```python
from build123d import *

# Parameters (mm, degrees)
SKETCH1_W           = 13.5
SKETCH1_H           = 29
BOSS_EXTRUDE1_DEPTH = 2
BOSS_EXTRUDE2_DEPTH = 56
BOSS_EXTRUDE3_DEPTH = 2
BOSS_EXTRUDE6_DEPTH = 23
SKETCH7_R           = 4.875
CUT_EXTRUDE2_DEPTH  = 6
BOSS_EXTRUDE7_REACH = 60
BOSS_EXTRUDE8_DEPTH = 6
CUT_EXTRUDE11_DEPTH = 5
SKETCH17_R          = 0.75
CUT_EXTRUDE13_DEPTH = 6
SKETCH18_R          = 6.425
CUT_EXTRUDE14_DEPTH = 6
SKETCH8_R           = 4.875
SKETCH8_R_2         = 2.775
CUT_EXTRUDE20_DEPTH = 20
SKETCH5_R           = 2.775
CUT_EXTRUDE21_DEPTH = 26
SKETCH19_R          = 2.775
CUT_EXTRUDE22_DEPTH = 26


with BuildPart() as part:
    # Sketch1 → Boss-Extrude1 (new body)
    with BuildSketch(Plane.XY):
        Polygon((23.484890655, 4.171572875), (0.484890655, 27.171572875), (0.484890655, -37.500000005), (23.484890655, -37.500000005), align=None)
        with Locations((11.635259587, -14.642279086)):
            Rectangle(SKETCH1_W, SKETCH1_H, mode=Mode.SUBTRACT)
        Polygon((23.484890655, 4.171572875), (23.484890655, -37.500000005), (0.484890655, -37.500000005), (0.484890655, -39.5), (25.484890655, -39.5), (25.484890655, 5), (0.484890655, 30), (0.484890655, 27.171572875), align=None)
    extrude(amount=BOSS_EXTRUDE1_DEPTH)

    # Sketch2 → Boss-Extrude2 (add)
    with BuildSketch(Plane.XY.offset(2)):
        Polygon((23.484890655, -37.500000005), (0.484890655, -37.500000005), (0.484890655, -39.5), (25.484890655, -39.5), (25.484890655, 5), (0.484890655, 30), (0.484890655, 27.171572875), (23.484890655, 4.171572875), align=None)
    extrude(amount=BOSS_EXTRUDE2_DEPTH)

    # Sketch3 → Boss-Extrude3 (add)
    with BuildSketch(Plane.XY.offset(58)):
        Polygon((25.484890655, 5), (0.484890655, 30), (0.484890655, -39.5), (25.484890655, -39.5), align=None)
    extrude(amount=BOSS_EXTRUDE3_DEPTH)

    # Sketch6 → Boss-Extrude6 (add)
    with BuildSketch(Plane.ZY.offset(-23.484890655)):
        with BuildLine():
            Line((37, -37.500000005), (37, -31.5))
            ThreePointArc((37, -31.5), (30, -24.5), (23, -31.5))
            Line((23, -31.5), (23, -37.500000005))
            Line((23, -37.500000005), (37, -37.500000005))
        make_face()
    extrude(amount=BOSS_EXTRUDE6_DEPTH)

    # Sketch7 → Cut-Extrude2 (cut)
    with BuildSketch(Plane(origin=(25.484890655, 0, 0), x_dir=(0, 0, -1), z_dir=(1, 0, 0))):
        with Locations((-30, -31.5)):
            Circle(SKETCH7_R)
    extrude(amount=-CUT_EXTRUDE2_DEPTH, mode=Mode.SUBTRACT)

    # Sketch9 → Boss-Extrude7 (add, up to next)
    with BuildSketch(Plane.XY.offset(2), mode=Mode.PRIVATE) as boss_extrude7_sk1:
        Polygon((0.484890655, 27.171572875), (17.541784111, 10.114679419), (0.484890655, 10.114679419), align=None)
    boss_extrude7_tool1 = extrude(boss_extrude7_sk1.sketch, amount=BOSS_EXTRUDE7_REACH, mode=Mode.PRIVATE) - part.part
    add(boss_extrude7_tool1.solids().sort_by_distance((6.170522, 15.800311, 2))[0])

    # Sketch14 → Boss-Extrude8 (add)
    with BuildSketch(Plane(origin=(0, 0, 58), x_dir=(-1, 0, 0), z_dir=(0, 0, -1))):
        Polygon((-17.541784111, 10.114679419), (-0.484890655, 10.114679419), (-0.484890655, -37.500000005), (-23.484890655, -37.500000005), (-23.484890655, 4.171572875), align=None)
    extrude(amount=BOSS_EXTRUDE8_DEPTH)

    # Sketch15 → Cut-Extrude11 (cut)
    with BuildSketch(Plane.XY.offset(60)):
        with BuildLine():
            Line((9.606797633, -3.100018288), (5.995686967, -10.67958818))
            ThreePointArc((5.995686967, -10.67958818), (5.371033475, -13.44302904), (5.995686967, -16.206469901))
            Line((5.995686967, -16.206469901), (9.606797633, -23.786039793))
            ThreePointArc((9.606797633, -23.786039793), (11.796033475, -25.16802904), (13.985269316, -23.786039793))
            Line((13.985269316, -23.786039793), (17.596379983, -16.206469901))
            ThreePointArc((17.596379983, -16.206469901), (18.221033475, -13.44302904), (17.596379983, -10.67958818))
            Line((17.596379983, -10.67958818), (13.985269316, -3.100018288))
            ThreePointArc((13.985269316, -3.100018288), (11.796033475, -1.71802904), (9.606797633, -3.100018288))
        make_face()
    extrude(amount=-CUT_EXTRUDE11_DEPTH, mode=Mode.SUBTRACT)

    # Sketch17 → Cut-Extrude13 (cut)
    with BuildSketch(Plane.XY.offset(55)):
        with Locations((11.796033475, -4.14302904)):
            Circle(SKETCH17_R)
        with Locations((11.796033475, -22.74302904)):
            Circle(SKETCH17_R)
    extrude(amount=-CUT_EXTRUDE13_DEPTH, mode=Mode.SUBTRACT)

    # Sketch18 → Cut-Extrude14 (cut)
    with BuildSketch(Plane.XY.offset(55)):
        with Locations((11.796033475, -13.44302904)):
            Circle(SKETCH18_R)
    extrude(amount=-CUT_EXTRUDE14_DEPTH, mode=Mode.SUBTRACT)

    # Sketch8 → Cut-Extrude20 (cut)
    with BuildSketch(Plane(origin=(25.484890655, 0, 0), x_dir=(0, 0, -1), z_dir=(1, 0, 0))):
        with Locations((-50, 18)):
            Circle(SKETCH8_R)
        with Locations((-50, 18)):
            Circle(SKETCH8_R_2, mode=Mode.SUBTRACT)
        with Locations((-10, 18)):
            Circle(SKETCH8_R)
        with Locations((-10, 18)):
            Circle(SKETCH8_R_2, mode=Mode.SUBTRACT)
    extrude(amount=-CUT_EXTRUDE20_DEPTH, mode=Mode.SUBTRACT)

    # Sketch5 → Cut-Extrude21 (cut, through all)
    with BuildSketch(Plane(origin=(25.484890655, 0, 0), x_dir=(0, 0, -1), z_dir=(1, 0, 0))):
        with Locations((-30, -31.5)):
            Circle(SKETCH5_R)
    extrude(amount=-CUT_EXTRUDE21_DEPTH, mode=Mode.SUBTRACT)

    # Sketch19 → Cut-Extrude22 (cut, through all)
    with BuildSketch(Plane(origin=(25.484890655, 0, 0), x_dir=(0, 0, -1), z_dir=(1, 0, 0))):
        with Locations((-50, 18)):
            Circle(SKETCH19_R)
        with Locations((-10, 18)):
            Circle(SKETCH19_R)
    extrude(amount=-CUT_EXTRUDE22_DEPTH, mode=Mode.SUBTRACT)


solid = part.part
```
The model under review builds one solid part; all positions refer to its coordinate system, in mm. A direction names the side the tool comes from. Round coordinates to 2 decimals unless told otherwise and drop trailing zeros. Loops run counter-clockwise (first coordinate to the right, second up) from the corner with the lowest first, then second, coordinate; pieces in that order, holes last. Notation, with made-up numbers: (82, -29.5) -> (110, -29.5) arc R8 ccw to (110, -23.5) -> close; hole circle Ø4 at (30.25, 2.5). An arc over 180 degrees is marked (long way). Answer in a Markdown table with one row per item.
1) Consider section C-C, the plane z = 39. Write out the cut boundary in (x, y), plus the area to 3 significant figures.
Taken from the geometry:
| item | result |
|---|---|
| outline | (0.48, -39.5) -> (25.48, -39.5) -> (25.48, 5) -> (0.48, 30) -> (0.48, 10.11) -> (17.54, 10.11) -> (23.48, 4.17) -> (23.48, -37.5) -> (0.48, -37.5) -> close |
| area | 348 mm² |
2) Consider section B-B, the plane y = -21. Write out the cut boundary in (x, z).
Taken from the geometry:
| item | result |
|---|---|
| outline | (0.48, 0) -> (4.89, 0) -> (4.89, 2) -> (0.48, 2) -> close; (0.48, 52) -> (23.48, 52) -> (23.48, 2) -> (18.39, 2) -> (18.39, 0) -> (25.48, 0) -> (25.48, 60) -> (15.31, 60) -> (15.31, 55) -> (8.28, 55) -> (8.28, 60) -> (0.48, 60) -> close |
3) Consider section D-D, the plane y = 18. Write out the cut boundary in (x, z) (3 decimals).
Taken from the geometry:
| item | result |
|---|---|
| outline | (0.485, 0) -> (12.485, 0) -> (12.485, 5.125) -> (5.485, 5.125) -> (5.485, 7.225) -> (0.485, 7.225) -> close; (0.485, 12.775) -> (5.485, 12.775) -> (5.485, 14.875) -> (12.485, 14.875) -> (12.485, 45.125) -> (5.485, 45.125) -> (5.485, 47.225) -> (0.485, 47.225) -> close; (0.485, 52.775) -> (5.485, 52.775) -> (5.485, 54.875) -> (12.485, 54.875) -> (12.485, 60) -> (0.485, 60) -> close |
4) Wall thickness on line 1 along Y through (x, z) = (11, 10) (3 decimals); line 2 along Z through (x, y) = (21.25, -30.5); line 3 along Y through (x, z) = (12.5, 30) (3 decimals): over which ranges is each line inside the solid? List them lowest first.
Taken from the geometry:
| item | result |
|---|---|
| line 1 | y = -39.5 to -37.5, 10.115 to 13.125 |
| line 2 | z = 0 to 2, 23.07 to 25.23, 34.77 to 36.93, 52 to 60 |
| line 3 | y = -39.5 to -34.275, -28.725 to -24.5, 10.115 to 17.985 |
5) Tool access review of faces 1 (the cylindrical face through (12.15, -24.5, 30.15)), 2 (the cylindrical face through (3.02, 15.29, 10.6)), 3 (the cylindrical face through (10.19, 13.24, 51.06)), 4 (the flat face through (12, -29.142, 1)), 5 (the flat face through (15.766, -20.049, 57.535)): name each direction out of +Z, -Z, +X, -X, +Y, -Y from which nothing blocks a thin tool from reaching the whole face with its end or side.
Taken from the geometry:
| item | result |
|---|---|
| face 1 | -X |
| face 2 | +X, -X |
| face 3 | +X |
| face 4 | -Z |
| face 5 | +Z |
6) For pin 1 Ø2 at (x, y) = (22.5, 11) entering from +Z; pin 2 Ø12 at (x, z) = (16.5, 43) entering from +Y; pin 3 Ø6.5 at (x, z) = (13, 10) entering from +Y; pin 4 Ø6 at (y, z) = (-7, 19.5) entering from -X, all flat-tipped, find the tip position at first contact; note any pin that passes through.
Taken from the geometry:
| item | result |
|---|---|
| pin 1 | passes through |
| pin 2 | stops at y = 19.98 |
| pin 3 | stops at y = 14.37 |
| pin 4 | stops at x = 23.48 |
7) Draft analysis for pull direction X (two halves, no side actions). For faces 6 (the cylindrical face through (12.511, -22.518, 53.521)), 7 (the flat face through (12, -37.5, 12)), 8 (the flat face through (5.485, 15.9, 7.9)), state which applies: pulls with the +X half, pulls with the -X half, needs draft (parallel to the pull), parting line crosses it, or undercut.
Taken from the geometry:
| item | result |
|---|---|
| face 6 | undercut |
| face 7 | needs draft |
| face 8 | pulls with the +X half |
8) Consider section A-A, the plane z = 30. Write out the cut boundary in (x, y) (3 decimals), plus the area to 3 significant figures.
Taken from the geometry:
| item | result |
|---|---|
| outline | (0.485, -39.5) -> (25.485, -39.5) -> (25.485, -36.375) -> (19.485, -36.375) -> (19.485, -34.275) -> (0.485, -34.275) -> close; (0.485, -28.725) -> (19.485, -28.725) -> (19.485, -26.625) -> (25.485, -26.625) -> (25.485, 5) -> (0.485, 30) -> (0.485, 10.115) -> (17.542, 10.115) -> (23.485, 4.172) -> (23.485, -24.5) -> (0.485, -24.5) -> close |
| area | 483 mm² |
